from build123d import *

# Parameters (mm, degrees)
F0_R     = 30
F0_R_2   = 5
F0_R_3   = 8.5
F1_DEPTH = 10


with BuildPart() as f1:
    # F0 (on Front) → F1 (new body)
    with BuildSketch(Plane.XZ):
        Circle(F0_R)
        with Locations((-16.263456, -16.263456)):
            Circle(F0_R_2, mode=Mode.SUBTRACT)
        with Locations((16.263456, -16.263456)):
            Circle(F0_R_2, mode=Mode.SUBTRACT)
        with Locations((0, -15)):
            Circle(F0_R_3, mode=Mode.SUBTRACT)
        with BuildLine():
            ThreePointArc((3.24037, 2.75), (0, -4.25), (-3.24037, 2.75))
            Line((-3.24037, 2.75), (3.24037, 2.75))
        make_face(mode=Mode.SUBTRACT)
        with Locations((-15, 0)):
            Circle(F0_R_3, mode=Mode.SUBTRACT)
        with Locations((-16.263456, 16.263456)):
            Circle(F0_R_2, mode=Mode.SUBTRACT)
        with Locations((15, 0)):
            Circle(F0_R_3, mode=Mode.SUBTRACT)
        with Locations((0, 15)):
            Circle(F0_R_3, mode=Mode.SUBTRACT)
        with Locations((16.263456, 16.263456)):
            Circle(F0_R_2, mode=Mode.SUBTRACT)
    extrude(amount=F1_DEPTH)


solid = f1.part
For this review, take the finished solid that the model builds, in its own axes (mm). A direction names the side the tool comes from. Give positions to 0.01 mm unless a question says otherwise; leave off trailing zeros. Loops run counter-clockwise (first coordinate to the right, second up) from the corner with the lowest first, then second, coordinate; pieces in that order, holes last.
Item 1: Tool access review of faces 4 (the flat face through (2, -10, -4)), 5 (the flat face through (0, -5, 2.75)): name each direction out of +Z, -Z, +X, -X, +Y, -Y from which nothing blocks a thin tool from reaching the whole face with its end or side.
Item 2: Insertion check: pin 1 (5 mm diameter, centred on x = 0.5, y = -6, fed in from -Z); pin 2 (2 mm diameter, centred on x = 15, y = -5, fed in from -Z); pin 3 (1.5 mm diameter, centred on y = -2, z = 17, fed in from +X). Each pin has a flat end and moves straight along its axis. Give the tip position at first contact, or say it passes through.
Item 3: Take a section at A-A, the plane x = 18. State the section outline as (y, z) points, and give its area (3 significant figures).
Item 4: Draft analysis for pull direction X (two halves, no side actions). For faces 1 (the cylindrical face through (-1.84, -4.93, -23.3)), 2 (the cylindrical face through (-29.97, -4.93, 1.32)), 3 (the flat face through (2, 0, -4)), state which applies: +X half, -X half, draft (parallel to the pull), parting line (faces both ways), or undercut.
Item 5: Take a section at C-C, the plane x = -10. State the section outline as (y, z) points.
Item 6: For line 1 along Z through (x, y) = (0, -2.25); line 2 along Z through (x, y) = (-15, -3); line 3 along X through (y, z) = (-1.25, -18), list the stretches that pass through material, from the lowest coordinate up.
Item 7: Take a section at B-B, the plane z = -15. State the section outline as (x, y) points.
Item 8: Take a section at D-D, the plane y = -6.5. Give the number of separate pieces and of enclosed holes in the cut face, and give its area (3 significant figures).
Calculated:
1. face 4: +Z, -Z, +X, -X, -Y
1. face 5: +Y, -Y
2. pin 1: stops at z = -30
2. pin 2: stops at z = -26.53
2. pin 3: stops at x = 25.22
3. outline: (-10, -24) - (0, -24) - (0, -20.95) - (-10, -20.95) - close; (-10, -11.57) - (0, -11.57) - (0, -7.95) - (-10, -7.95) - close; (-10, 7.95) - (0, 7.95) - (0, 11.57) - (-10, 11.57) - close; (-10, 20.95) - (0, 20.95) - (0, 24) - (-10, 24) - close
3. area: 133 mm2
4. face 1: undercut
4. face 2: parting line
4. face 3: draft
5. outline: (-10, -28.28) - (0, -28.28) - (0, -6.87) - (-10, -6.87) - close; (-10, 6.87) - (0, 6.87) - (0, 28.28) - (-10, 28.28) - close
6. line 1: z = -30 to -23.5, -6.5 to -4.25, 2.75 to 6.5, 23.5 to 30
6. line 2: z = -25.98 to -21.1, -11.43 to -8.5, 8.5 to 11.43, 21.1 to 25.98
6. line 3: x = -24 to -20.95, -11.57 to -7.95, 7.95 to 11.57, 20.95 to 24
7. outline: (-25.98, -10) - (-21.1, -10) - (-21.1, 0) - (-25.98, 0) - close; (-11.43, -10) - (-8.5, -10) - (-8.5, 0) - (-11.43, 0) - close; (8.5, -10) - (11.43, -10) - (11.43, 0) - (8.5, 0) - close; (21.1, -10) - (25.98, -10) - (25.98, 0) - (21.1, 0) - close
8. separate pieces: 1
8. enclosed holes: 9
8. area: 1,560 mm2
